For this review, take the finished solid that the model builds, in its own axes (mm). A direction names the side the tool comes from. Give positions to 0.01 mm unless a question says otherwise; leave off trailing zeros. Order: outer loops, then holes, each group sorted by start corner. A loop starts at its lowest first (then second) coordinate and runs counter-clockwise, first axis right, second up. Notation, with made-up numbers: (-16.5, 4) -> (37.5, 4) arc R22 ccw to (37.5, 25) -> close; hole circle Ø2 at (-34, -14). An arc over 180 degrees is marked (long way). Return JSON: item names as keys, results as strings. Group by question number.
1) Add section C-C (x = 46.5). State how many separate pieces and enclosed holes the cut face has, then the cut area to 3 significant figures.
2) Insertion check: P1, Ø6, axis at x = 29.5, y = -13, coming from the -Z side; P2, Ø4, axis at x = 0, y = -24.5, coming from the -Z side; P3, Ø5, axis at x = 1.5, y = -19.5, coming from the +Z side. Each pin has a flat end and moves straight along its axis. Give the tip position at first contact, or say it passes through.
3) To check wall thickness, follow line 1 along Y through (x, z) = (-46.5, 1.2); line 2 along X through (y, z) = (-24, 13); line 3 along X through (y, z) = (1, 2.5). State the ranges of each line that lie inside material, in increasing order.
4) Add section D-D (y = -12). Give the boundary of the cut face in (x, z).
5) Add section A-A (z = 3.75). Give the boundary of the cut face in (x, y).
6) The part is to be moulded in two halves that separate along X. For faces 1 (the face through (51, 5, 5)), 2 (the face through (9.52, -22.6, 11.68)), 3 (the face through (-47, 25, 2)), say which applies: released by +X, released by -X, zero draft, split by the parting line, or undercut.
7) For faces 4 (the face through (11, -20, 16)), 5 (the face through (9.736, -27, 4)), 6 (the face through (45.39, -26.49, 2.46)), 7 (the face through (49, 30, 2)), 8 (the face through (44, 28, 2)), list the 3-axis set-ups (+Z, -Z, +X, -X, +Y, -Y) from which the entire face can be reached by the end or side of a thin tool; tool diameter is ignored.
8) Add section B-B (y = 5.5). Give the boundary of the cut face in (x, z).
from build123d import *

# Parameters (mm, degrees)
SKETCH3_R           = 1.5
BOSS_EXTRUDE2_DEPTH = 5
BOSS_EXTRUDE3_DEPTH = 108
CUT_EXTRUDE1_REACH  = 53.226
SKETCH5_R           = 1.6
CUT_EXTRUDE2_REACH  = 53.226
SKETCH6_W           = 3
SKETCH6_H           = 10
SKETCH7_W           = 19.472559222
SKETCH7_H           = 21.170747527
CUT_EXTRUDE3_DEPTH  = 61


with BuildPart() as part:
    # Sketch3 → Boss-Extrude2 (new body)
    with BuildSketch(Plane.XY):
        Polygon((-49, 25), (-44, 25), (-44, 30), (-49, 30), (-54, 30), (-54, 25), (-54, -25), (-54, -30), (-49, -30), (-44, -30), (44, -30), (49, -30), (54, -30), (54, -25), (54, 25), (54, 30), (49, 30), (44, 30), (44, 25), (49, 25), (49, -25), (44, -25), (-44, -25), (-49, -25), align=None)
        with BuildLine():
            ThreePointArc((-46.5, -26), (-45.439339828, -26.439339828), (-45, -27.5))
            ThreePointArc((-45, -27.5), (-47.560660172, -28.560660172), (-46.5, -26))
        make_face(mode=Mode.SUBTRACT)
        with Locations((46.5, -27.5)):
            Circle(SKETCH3_R, mode=Mode.SUBTRACT)
        with BuildLine():
            ThreePointArc((-45, 27.5), (-45.439339828, 26.439339828), (-46.5, 26))
            ThreePointArc((-46.5, 26), (-47.560660172, 28.560660172), (-45, 27.5))
        make_face(mode=Mode.SUBTRACT)
        with Locations((46.5, 27.5)):
            Circle(SKETCH3_R, mode=Mode.SUBTRACT)
    extrude(amount=BOSS_EXTRUDE2_DEPTH)

    # Sketch4 → Boss-Extrude3 (add)
    with BuildSketch(Plane(origin=(54, 0, 0), x_dir=(0, 0, -1), z_dir=(1, 0, 0))):
        Polygon((-5, -30), (-5, -25.001535135), (-26.363936199, -9.214733726), (-26.363936199, -14.213198591), align=None)
    extrude(amount=-BOSS_EXTRUDE3_DEPTH)

    # Sketch5 → Cut-Extrude1 (cut, up to next)
    with BuildSketch(Plane(origin=(0, -21.794194287, 16.104739027), x_dir=(-1, 0, 0), z_dir=(0, -0.804246926, 0.594295282)), mode=Mode.PRIVATE) as cut_extrude1_sk1:
        with Locations((47, -7.13269846)):
            Circle(SKETCH5_R)
    cut_extrude1_tool1 = extrude(cut_extrude1_sk1.sketch, amount=-CUT_EXTRUDE1_REACH, mode=Mode.PRIVATE) & part.part
    add(cut_extrude1_tool1.solids().sort_by_distance((-47, -17.555265, 21.84119))[0], mode=Mode.SUBTRACT)
    # Sketch5 → Cut-Extrude1 (cut, up to next)
    with BuildSketch(Plane(origin=(0, -21.794194287, 16.104739027), x_dir=(-1, 0, 0), z_dir=(0, -0.804246926, 0.594295282)), mode=Mode.PRIVATE) as cut_extrude1_sk2:
        with Locations((-47, -7.13269846)):
            Circle(SKETCH5_R)
    cut_extrude1_tool2 = extrude(cut_extrude1_sk2.sketch, amount=-CUT_EXTRUDE1_REACH, mode=Mode.PRIVATE) & part.part
    add(cut_extrude1_tool2.solids().sort_by_distance((47, -17.555265, 21.84119))[0], mode=Mode.SUBTRACT)

    # Sketch6 → Cut-Extrude2 (cut, up to next)
    with BuildSketch(Plane(origin=(0, -21.794194287, 16.104739027), x_dir=(-1, 0, 0), z_dir=(0, -0.804246926, 0.594295282)), mode=Mode.PRIVATE) as cut_extrude2_sk1:
        with Locations((-9.5, -0.964147651)):
            Rectangle(SKETCH6_W, SKETCH6_H)
    cut_extrude2_tool1 = extrude(cut_extrude2_sk1.sketch, amount=-CUT_EXTRUDE2_REACH, mode=Mode.PRIVATE) & part.part
    add(cut_extrude2_tool1.solids().sort_by_distance((9.5, -21.221206, 16.880152))[0], mode=Mode.SUBTRACT)
    # Sketch6 → Cut-Extrude2 (cut, up to next)
    with BuildSketch(Plane(origin=(0, -21.794194287, 16.104739027), x_dir=(-1, 0, 0), z_dir=(0, -0.804246926, 0.594295282)), mode=Mode.PRIVATE) as cut_extrude2_sk2:
        with Locations((9.5, -0.964147651)):
            Rectangle(SKETCH6_W, SKETCH6_H)
    cut_extrude2_tool2 = extrude(cut_extrude2_sk2.sketch, amount=-CUT_EXTRUDE2_REACH, mode=Mode.PRIVATE) & part.part
    add(cut_extrude2_tool2.solids().sort_by_distance((-9.5, -21.221206, 16.880152))[0], mode=Mode.SUBTRACT)

    # Sketch7 → Cut-Extrude3 (cut, through all)
    with BuildSketch(Plane(origin=(0, -30, 0), x_dir=(-1, 0, 0), z_dir=(0, -1, 0))):
        with Locations((0, 2.554576853)):
            Rectangle(SKETCH7_W, SKETCH7_H)
    extrude(amount=-CUT_EXTRUDE3_DEPTH, mode=Mode.SUBTRACT)


solid = part.part
Evaluation:
{
 "1": {"separate pieces": "4", "enclosed holes": "0", "area": "115 mm^2"},
 "2": {"P1": "z = 17.18", "P2": "z = 8.03", "P3": "z = 22.59"},
 "3": {"line 1": "-30 to -29, -26 to -25, 25 to 26, 29 to 30", "line 2": "-54 to -11, -8 to 8, 11 to 54", "line 3": "-54 to -49, 49 to 54"},
 "4": {"outline": "(-54, 0) -> (-49, 0) -> (-49, 5) -> (-54, 5) -> close; (-54, 22.59) -> (54, 22.59) -> (54, 26.36) -> (-54, 26.36) -> close; (49, 0) -> (54, 0) -> (54, 5) -> (49, 5) -> close"},
 "5": {"outline": "(-54, -30) -> (-9.74, -30) -> (-9.74, -25) -> (-49, -25) -> (-49, 25) -> (-44, 25) -> (-44, 30) -> (-54, 30) -> close; (9.74, -30) -> (54, -30) -> (54, 30) -> (44, 30) -> (44, 25) -> (49, 25) -> (49, -25) -> (9.74, -25) -> close; hole circle Ø3 at (-46.5, -27.5); hole circle Ø3 at (-46.5, 27.5); hole circle Ø3 at (46.5, -27.5); hole circle Ø3 at (46.5, 27.5)"},
 "6": {"face 1": "zero draft", "face 2": "undercut", "face 3": "undercut"},
 "7": {"face 4": "none", "face 5": "-Z, +Y, -Y", "face 6": "-Z", "face 7": "+Z, -Z, +X, -X, +Y", "face 8": "+Z, -Z, +Y"},
 "8": {"outline": "(-54, 0) -> (-49, 0) -> (-49, 5) -> (-54, 5) -> close; (49, 0) -> (54, 0) -> (54, 5) -> (49, 5) -> close"}
}
